```python
from build123d import *

# Parameters (mm, degrees)
F0_W      = 127.8839372098
F0_H      = 94.8674269021
F1_DEPTH  = 3.81
F2_W      = 127.8839372098
F2_H      = 94.8674269021
F2_W_2    = 120.2639372098
F2_H_2    = 87.2474269021
F3_DEPTH  = 25.4
F5_DEPTH  = 25.4
F6_W      = 2.2098
F6_H      = 41.744076617
F7_DEPTH  = 25.4
F9_DEPTH  = 25.4
F11_DEPTH = 25.4
F12_W     = 2.2098
F12_H     = 17.600103577
F13_DEPTH = 25.4
F14_W     = 2.2098
F14_H     = 23.4836467081
F15_DEPTH = 25.4
F17_DEPTH = 25.4
F19_DEPTH = 25.4
F21_DEPTH = 9.652
F23_DEPTH = 6.3754
F25_DEPTH = 11.43
F27_DEPTH = 11.43
F29_DEPTH = 10.414


with BuildPart() as f1:
    # F0 (on Top) → F1 (new body)
    with BuildSketch(Plane.XY):
        with Locations((-7.0435199887, -0.3301631659)):
            Rectangle(F0_W, F0_H)
    extrude(amount=F1_DEPTH)

    # F2 (on face) → F3 (join)
    with BuildSketch(Plane.XY.offset(3.81)):
        with Locations((-7.0435199887, -0.3301631659)):
            Rectangle(F2_W, F2_H)
        with Locations((-7.0435199887, -0.3301631659)):
            Rectangle(F2_W_2, F2_H_2, mode=Mode.SUBTRACT)
    extrude(amount=F3_DEPTH)

    # F4 (on face) → F5 (join)
    with BuildSketch(Plane.XY.offset(3.81)):
        Polygon((-24.9860885936, -2.2098), (-24.9860885936, 0), (-24.9824896455, 0), (-24.9824896455, 43.2935502851), (-27.1835904568, 43.2935502851), (-27.1835904568, 0), (-67.1754885936, 0), (-67.1754885936, -2.2098), align=None)
    extrude(amount=F5_DEPTH)

    # F6 (on face) → F7 (join)
    with BuildSketch(Plane.XY.offset(3.81)):
        with Locations((-26.0909885936, -23.0818383085)):
            Rectangle(F6_W, F6_H)
    extrude(amount=F7_DEPTH)

    # F8 (on face) → F9 (join)
    with BuildSketch(Plane.XY.offset(3.81)):
        Polygon((0, 0), (0, -43.953876617), (2.2098, -43.953876617), (2.2098, -2.2098), (53.0884486163, -2.2098), (53.0884486163, 0), align=None)
    extrude(amount=F9_DEPTH)

    # F10 (on face) → F11 (join)
    with BuildSketch(Plane.XY.offset(3.81)):
        Polygon((0, 0), (-24.9824896455, 0), (-26.9634798169, 0), (-26.9634798169, -2.2098), (-24.9860885936, -2.2098), (0, -2.2098), align=None)
    extrude(amount=F11_DEPTH)

    # F12 (on face) → F13 (join)
    with BuildSketch(Plane.XY.offset(3.81)):
        with Locations((23.6661800568, 8.8000517885)):
            Rectangle(F12_W, F12_H)
        Polygon((22.5612800568, 19.809903577), (22.5612800568, 17.600103577), (24.7710800568, 17.600103577), (53.0884486163, 17.600103577), (53.0884486163, 19.809903577), align=None)
    extrude(amount=F13_DEPTH)

    # F14 (on face) → F15 (join)
    with BuildSketch(Plane.XY.offset(3.81)):
        Polygon((53.0884486163, 17.600103577), (53.0884486163, 19.809903577), (19.0482183198, 19.809903577), (16.8384183198, 19.809903577), (16.8384183198, 17.600103577), align=None)
        with Locations((17.9433183198, 31.551726931)):
            Rectangle(F14_W, F14_H)
    extrude(amount=F15_DEPTH)

    # F16 (on face) → F17 (cut)
    with BuildSketch(Plane(origin=(0, -43.953876617, 0), x_dir=(-1, 0, 0), z_dir=(0, 1, 0))):
        Polygon((8.1807011738, 22.1107043326), (8.1807011738, 3.81), (16.5439341217, 3.81), (16.5439341217, 22.1107043326), (16.5439341217, 31.9952704012), (8.1807011738, 31.9952704012), align=None)
    extrude(amount=-F17_DEPTH, mode=Mode.SUBTRACT)

    # F18 (on face) → F19 (cut)
    with BuildSketch(Plane(origin=(0, 0, 0), x_dir=(0, -1, 0), z_dir=(-1, 0, 0))):
        Polygon((10.1021090522, 23.6382391304), (10.1021090522, 3.81), (18.1610379368, 3.81), (18.1610379368, 23.6382391304), (18.1610379368, 31.1116781086), (10.1021090522, 31.1116781086), align=None)
    extrude(amount=-F19_DEPTH, mode=Mode.SUBTRACT)

    # F20 (on face) → F21 (cut)
    with BuildSketch(Plane(origin=(-27.1958885936, 0, 0), x_dir=(0, -1, 0), z_dir=(-1, 0, 0))):
        Polygon((11.8822744116, 20.1589465141), (11.8822744116, 3.81), (19.8594387621, 3.81), (19.8594387621, 20.1589465141), (19.8594387621, 31.4402878284), (11.8822744116, 31.4402878284), align=None)
    extrude(amount=-F21_DEPTH, mode=Mode.SUBTRACT)

    # F22 (on face) → F23 (cut)
    with BuildSketch(Plane(origin=(-27.1835904568, 0, 0), x_dir=(0, -1, 0), z_dir=(-1, 0, 0))):
        Polygon((-23.0946410447, 19.9922583997), (-23.0946410447, 3.81), (-14.3088679761, 3.81), (-14.3088679761, 19.9922583997), (-14.3088679761, 32.4732325971), (-23.0946410447, 32.4732325971), align=None)
    extrude(amount=-F23_DEPTH, mode=Mode.SUBTRACT)

    # F24 (on face) → F25 (cut)
    with BuildSketch(Plane(origin=(22.5612800568, 0, 0), x_dir=(0, -1, 0), z_dir=(-1, 0, 0))):
        Polygon((-10.9547926113, 22.2612097859), (-10.9547926113, 3.81), (-3.4168059938, 3.81), (-3.4168059938, 22.2612097859), (-3.4168059938, 32.5798727572), (-10.9547926113, 32.5798727572), align=None)
    extrude(amount=-F25_DEPTH, mode=Mode.SUBTRACT)

    # F26 (on face) → F27 (cut)
    with BuildSketch(Plane.XZ.offset(-17.600103577)):
        Polygon((36.4499650896, 21.9316985458), (36.4499650896, 3.81), (41.7222119868, 3.81), (41.7222119868, 21.2429128587), (41.7222119868, 21.9316985458), (41.7222119868, 34.7188301384), (36.4499650896, 34.7188301384), align=None)
    extrude(amount=-F27_DEPTH, mode=Mode.SUBTRACT)

    # F28 (on face) → F29 (cut)
    with BuildSketch(Plane.XZ.offset(2.2098)):
        Polygon((-14.7642167285, 18.1317012757), (-14.7642167285, 3.81), (-8.2613723353, 3.81), (-8.2613723353, 18.1317012757), (-8.2613723353, 34.8567925394), (-14.7642167285, 34.8567925394), align=None)
    extrude(amount=-F29_DEPTH, mode=Mode.SUBTRACT)


solid = f1.part
```
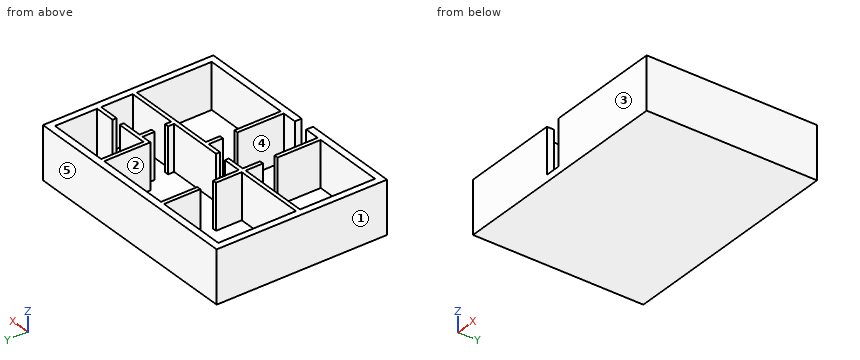
Geometry check sheet. Reference: the model listing, model coordinates, mm. Face numbers are marked on the shaded views. A direction names the side the tool comes from. Coordinates: 2 decimals unless noted, no trailing zeros. Order: outer loops, then holes, each group sorted by start corner. A loop starts at its lowest first (then second) coordinate and runs counter-clockwise, first axis right, second up. Notation, with made-up numbers: M 46,-25 L 69,-25 A22 ccw 69,-10 Z; hole C 49,83.5 d6. An arc over 180 degrees is marked long. Answer as a JSON object with one key per item and string values.
Q1. Cross-section at B-B on x = -46. Record the cut outline in (y, z), and give its area (3 significant figures).
Results are:
{"outline": "M -47.76,0 L 47.1,0 L 47.1,29.21 L 43.29,29.21 L 43.29,3.81 L 0,3.81 L 0,29.21 L -2.21,29.21 L -2.21,3.81 L -43.95,3.81 L -43.95,29.21 L -47.76,29.21 Z", "area": "611 mm²"}
Q2. Cross-section at C-C on x = 33.5. Record the cut outline in (y, z), and give its area (3 significant figures).
Results are:
{"outline": "M -47.76,0 L 47.1,0 L 47.1,29.21 L 43.29,29.21 L 43.29,3.81 L 19.81,3.81 L 19.81,29.21 L 17.6,29.21 L 17.6,3.81 L 0,3.81 L 0,29.21 L -2.21,29.21 L -2.21,3.81 L -43.95,3.81 L -43.95,29.21 L -47.76,29.21 Z", "area": "667 mm²"}
Q3. Tool access check on the marked faces 4 and 5. Record the directions out of +Z, -Z, +X, -X, +Y, -Y that give a thin tool (end or side, any length) a straight path to the whole face; none if there is none.
Results are:
{"face 4": "+Z", "face 5": "+Z, -Z, +X, -X, +Y"}
Q4. Release check for a two-part mould opening along X. For the marked faces 1, 2 and 3 record: released by +X, released by -X, zero draft, split by the parting line, or undercut.
Results are:
{"face 1": "released by -X", "face 2": "undercut", "face 3": "zero draft"}
Q5. Cross-section at A-A on y = -28. Record the cut outline in (x, z), and give its area (3 significant figures).
Results are:
{"outline": "M -70.99,0 L 56.9,0 L 56.9,29.21 L 53.09,29.21 L 53.09,3.81 L 2.21,3.81 L 2.21,29.21 L 0,29.21 L 0,3.81 L -24.99,3.81 L -24.99,29.21 L -27.2,29.21 L -27.2,3.81 L -67.18,3.81 L -67.18,29.21 L -70.99,29.21 Z", "area": "793 mm²"}
Q6. Cross-section at D-D on y = -16. Record the cut outline in (x, z), and give its area (3 significant figures).
Results are:
{"outline": "M -70.99,0 L 56.9,0 L 56.9,29.21 L 53.09,29.21 L 53.09,3.81 L -67.18,3.81 L -67.18,29.21 L -70.99,29.21 Z", "area": "681 mm²"}
Q7. Scan lines: line 1 (Y direction, x = 41, z = 20.75); line 2 (X direction, y = 23.5, z = 8.75); line 3 (X direction, y = -21.5, z = 22). Record each from-to range of solid material in increasing order.
Results are:
{"line 1": "y = -47.76 to -43.95, -2.21 to 0, 43.29 to 47.1", "line 2": "x = -70.99 to -67.18, -27.18 to -24.98, 16.84 to 19.05, 53.09 to 56.9", "line 3": "x = -70.99 to -67.18, -27.2 to -24.99, 0 to 2.21, 53.09 to 56.9"}
